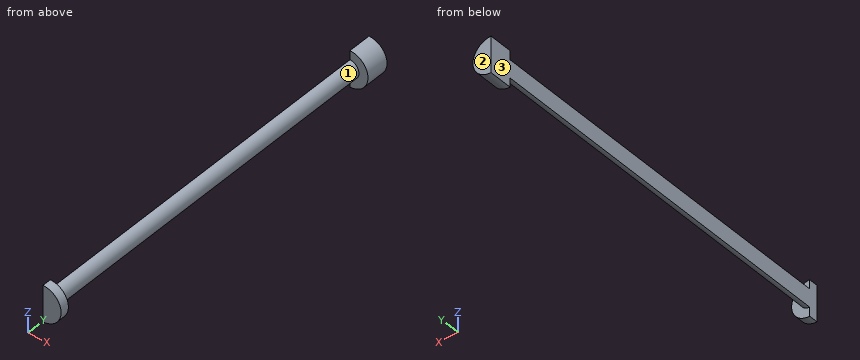
Autodesk Inventor part; units mm, degrees
ref_plane "YZ Plane" through (0, 0, 0) normal (1, 0, 0) x (0, 1, 0)
ref_plane "XZ Plane" through (0, 0, 0) normal (0, 1, 0) x (-1, 0, 0)
ref_plane "XY Plane" through (0, 0, 0) normal (0, 0, 1) x (1, 0, 0)
sketch "Sketch1" plane through (0, 0, 0) normal (0, 0, 1) x (1, 0, 0)
  line L0 (0, 0) -> (2.5, 0)
  line L1 (2.5, 0) -> (2.5, 107.3)
  line L2 (2.5, 107.3) -> (0, 107.3)
  line L3 (0, 107.3) -> (0, 0)
  line L4 (0, 107.3) -> (5, 107.3)
  line L5 (5, 107.3) -> (5, 104.8)
  line L6 (5, 104.8) -> (0, 104.8)
  line L7 (0, 104.8) -> (0, 107.3)
  line L8 (0, 0) -> (5, 0)
  line L9 (5, 0) -> (5, 2.5)
  line L10 (5, 2.5) -> (0, 2.5)
  line L11 (0, 2.5) -> (0, 0)
  point P0 (2.5, 2.5)
  point P1 (2.5, 104.8)
  dimension "d0" = 2.5
  dimension "d1" = 107.3
  dimension "d2" = 5
  dimension "d3" = 2.5
  dimension "d4" = 5
  dimension "d5" = 2.5
revolve "Revolution1" add sketch "Sketch1" angle 360 about axis through (0, 107.3, 0) along (0, -1, 0)
sketch "Sketch4" plane through (0, 107.3, 0) normal (0, 1, 0) x (1, 0, 0)
  circle A0 centre (0, 0) radius 5
  line L0 (0, -5) -> (0, 5)
  arc A1 (0, 5) -> (0, -5) centre (0, 0) ccw
extrude "Extrusion3" cut sketch "Sketch4" against normal through all contours L0 A0 picked at (-0.7745, -1.4758)
sketch "Sketch5" plane through (0, 107.3, 0) normal (0, 1, 0) x (1, 0, 0)
  arc A0 (0, -5) -> (0, 5) centre (0, 0) ccw
  line L0 (0, -5) -> (0, 5)
extrude "Extrusion4" add sketch "Sketch5" along normal blind 4
properties part number "Rod"
Geometry: final body of the model. Coordinates: model frame, mm. Face numbers are marked on the shaded views. Give positions to 0.01 mm unless a question says otherwise; leave off trailing zeros. Order: outer loops, then holes, each group sorted by start corner. A loop starts at its lowest first (then second) coordinate and runs counter-clockwise, first axis right, second up. Notation, with made-up numbers: M -20,13 L 24,13 A24 cw 24,45 Z; hole C 20,25.25 d9. An arc over 180 degrees is marked long. Answer as CSV lines item,"result". Start each with the question number.
1) Cut plane A-A (x = 3.4). Output: boundary loops of the cut face in (y, z).
2) Cut plane B-B (z = 0). Output: boundary loops of the cut face in (x, y), then the cut area to 3 significant figures.
3) Mould query, pull axis Y, two halves, no side actions, for the marked faces 1, 2 and 3. Classes: +Y half, -Y half, draft (parallel to the pull), parting line (faces both ways), or undercut.
4) First-contact query: P1, Ø2, axis at y = 80.5, z = 4, coming from the +X side; P2, Ø3, axis at y = 63.5, z = 0, coming from the -X side; P3, Ø3, axis at x = 3, y = 97, coming from the +Z side. Flat tips, straight axial feed; report the tip coordinate or a pass-through.
5) Cut plane C-C (y = 99). Output: boundary loops of the cut face in (x, z), then the cut area to 3 significant figures.
6) Line query: line 1 (Y direction, x = 4, z = -2); line 2 (Z direction, x = 0.3, y = 56); line 3 (X direction, y = 54, z = 1.75). Output: solid intervals per line, ascending. Write a range as from..to.
Findings below:
1,outline,"M 0,-3.67 L 2.5,-3.67 L 2.5,3.67 L 0,3.67 Z; M 104.8,-3.67 L 111.3,-3.67 L 111.3,3.67 L 104.8,3.67 Z"
2,outline,"M 0,0 L 5,0 L 5,2.5 L 2.5,2.5 L 2.5,104.8 L 5,104.8 L 5,111.3 L 0,111.3 Z"
2,area,"301 mm²"
3,face 1,"undercut"
3,face 2,"+Y half"
3,face 3,"draft"
4,P1,"passes through"
4,P2,"stops at x = 0"
4,P3,"stops at z = 2"
5,outline,"M 0,-2.5 A2.5 ccw 0,2.5 Z"
5,area,"9.82 mm²"
6,line 1,"y = 0..2.5, 104.8..111.3"
6,line 2,"z = -2.48..2.48"
6,line 3,"x = 0..1.79"
